from build123d import *

# Parameters (mm, degrees)
BOSS_EXTRUDE1_DEPTH = 210
SKETCH3_R           = 70
BOSS_EXTRUDE2_DEPTH = 20
BOSS_EXTRUDE2_TAPER = 25
SKETCH4_R           = 60.673846837
BOSS_EXTRUDE3_DEPTH = 20
CHAMFER1_SIZE       = 3.5
FILLET1_R           = 7
FILLET2_R           = 5


with BuildPart() as part:
    # Sketch2 → Boss-Extrude1 (new body)
    with BuildSketch(Plane.XY):
        Polygon((0, 0), (55, 0), (55, 10), (40, 10), (40, 20), (100, 20), (100, 10), (85, 10), (85, 0), (140, 0), (140, 10), (120, 10), (120, 20), (175, 20), (175, 80), (-35, 80), (-35, 20), (20, 20), (20, 10), (0, 10), align=None)
    extrude(amount=BOSS_EXTRUDE1_DEPTH)

    # Sketch3 → Boss-Extrude2 (add)
    with BuildSketch(Plane(origin=(0, 80, 0), x_dir=(1, 0, 0), z_dir=(0, 1, 0))):
        with Locations((70, -105)):
            Circle(SKETCH3_R)
    extrude(amount=BOSS_EXTRUDE2_DEPTH, taper=BOSS_EXTRUDE2_TAPER)

    # Sketch4 → Boss-Extrude3 (add)
    with BuildSketch(Plane(origin=(0, 100, 0), x_dir=(1, 0, 0), z_dir=(0, 1, 0))):
        with Locations(Location((70, -105, 0), (0, 0, 180))):
            Circle(SKETCH4_R)
    extrude(amount=BOSS_EXTRUDE3_DEPTH)

    # Chamfer1
    chamfer1_edges = [part.edges().sort_by_distance(p)[0] for p in [
        (-35, 50, 0),
        (175, 50, 0),
        (175, 50, 210),
        (-35, 50, 210),
    ]]
    chamfer(chamfer1_edges, length=CHAMFER1_SIZE)

    # Fillet1
    fillet1_edges = [part.edges().sort_by_distance(p)[0] for p in [
        (0, 80, 105),
        (70, 100, 44.326153163),
    ]]
    fillet(fillet1_edges, radius=FILLET1_R)

    # Fillet2
    # the kernel refuses this fillet: 5 mm, written as the material it takes off along each edge
    with BuildSketch(Plane(origin=(-35, 80, -9), x_dir=(1, 0, 0), z_dir=(0, 0, 1)), Plane(origin=(184, 80, 0), x_dir=(0, 0, 1), z_dir=(-1, 0, 0))) as fillet2_piece_1:
        with BuildLine():
            CenterArc((FILLET2_R, -FILLET2_R), FILLET2_R, 90, 90)
            Line((0, -FILLET2_R), (0, 0))
            Line((0, 0), (FILLET2_R, 0))
        make_face()
    extrude(amount=228, mode=Mode.SUBTRACT)
    with BuildSketch(Plane(origin=(175, 80, -9), x_dir=(-1, 0, 0), z_dir=(0, 0, 1)), Plane(origin=(184, 80, 210), x_dir=(0, 0, -1), z_dir=(-1, 0, 0))) as fillet2_piece_2:
        with BuildLine():
            CenterArc((FILLET2_R, FILLET2_R), FILLET2_R, 180, 90)
            Line((0, FILLET2_R), (0, 0))
            Line((0, 0), (FILLET2_R, 0))
        make_face()
    extrude(amount=228, mode=Mode.SUBTRACT)


solid = part.part
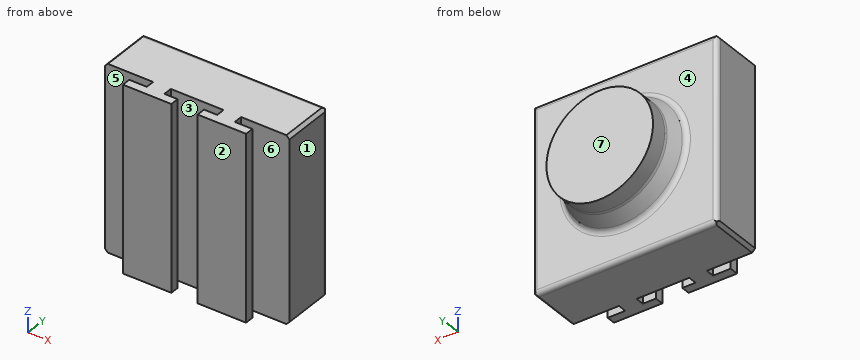
Geometry check sheet. Reference: the model listing, model coordinates, mm. Face numbers are marked on the shaded views. A direction names the side the tool comes from. Give positions to 0.01 mm unless a question says otherwise; leave off trailing zeros. Order: outer loops, then holes, each group sorted by start corner. A loop starts at its lowest first (then second) coordinate and runs counter-clockwise, first axis right, second up. Notation, with made-up numbers: (43.25, 70.5) - (82.25, 70.5) arc R17 ccw to (82.25, 80.5) - close; hole circle Ø1 at (42.25, 83). An arc over 180 degrees is marked (long way). Use one line per item in the form item = value.
1) Material ranges on probe 1 along X at (y, z) = (19, 108.5); probe 2 along Y at (x, z) = (11.5, 104); probe 3 along Y at (x, z) = (7.5, 114.5), recorded low to high. Write a range as from..to.
Working result:
probe_1 = 20..40, 100..120
probe_2 = 0..10, 20..120
probe_3 = 0..10, 20..94.54
2) Access from +Z, -Z, +X, -X, +Y, -Y to the whole of each face (thin tool, end or side, straight path). Record for the marked faces 4, 5, 6 and 7.
Working result:
face_4 = +Y
face_5 = +Z, -Z, -X
face_6 = +Z, -Z, +X
face_7 = +Z, -Z, +X, -X, +Y
3) Sectioned sample at B-B (z = 13). Record the boundary of the cut face in (x, y), and give its area (3 significant figures).
Working result:
outline = (-35, 20) - (20, 20) - (20, 10) - (0, 10) - (0, 0) - (55, 0) - (55, 10) - (40, 10) - (40, 20) - (100, 20) - (100, 10) - (85, 10) - (85, 0) - (140, 0) - (140, 10) - (120, 10) - (120, 20) - (175, 20) - (175, 75) arc R5 ccw to (170, 80) - (-30, 80) arc R5 ccw to (-35, 75) - close
area = 14,100 mm^2
4) Sectioned sample at A-A (y = 17). Record the boundary of the cut face in (x, z), and give its area (3 significant figures).
Working result:
outline = (20, 0) - (40, 0) - (40, 210) - (20, 210) - close; (100, 0) - (120, 0) - (120, 210) - (100, 210) - close
area = 8,400 mm^2
5) Draft check along X on the marked faces 1, 2 and 3. Enter one of: released by +X, released by -X, zero draft, split by the parting line, or undercut.
Working result:
face_1 = released by +X
face_2 = zero draft
face_3 = undercut
6) Depth check by flat-ended pin: pin 1 Ø11 at (y, z) = (6.5, 124.5) entering from -X; pin 2 Ø5 at (x, z) = (138, 175) entering from +Y; pin 3 Ø5 at (y, z) = (6, 88) entering from +X; pin 4 Ø16.5 at (x, z) = (142.5, 121.5) entering from -Y. Enter the tip coordinate at first touch or a pass-through.
Working result:
pin_1 = 0
pin_2 = 80
pin_3 = 140
pin_4 = 0
